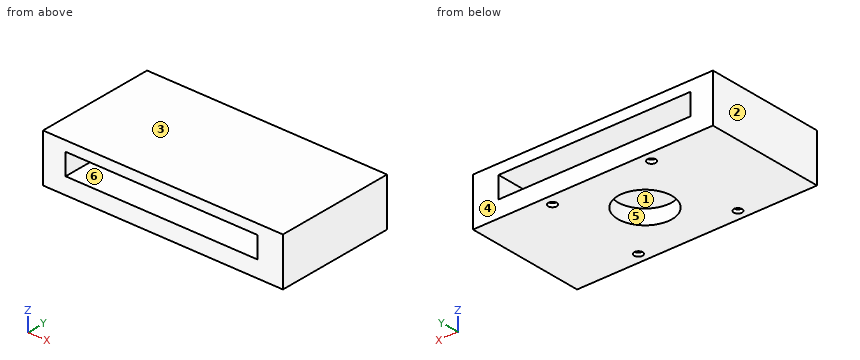
```python
from build123d import *

# Parameters (mm, degrees)
F0_W     = 2000
F0_H     = 425
F0_W_2   = 1598.0344712734
F0_H_2   = 178.1892329454
F1_DEPTH = 1000
F2_DEPTH = 25
F3_R     = 35
F4_DEPTH = 30
F5_R     = 225
F6_DEPTH = 122
F7_SCALE = 0.055


with BuildPart() as f1:
    # F0 (on Front) → F1 (new body)
    with BuildSketch(Plane.XZ):
        with Locations((-1000, 212.5)):
            Rectangle(F0_W, F0_H)
        with Locations((-1012.4687701464, 227.0783409476)):
            Rectangle(F0_W_2, F0_H_2, mode=Mode.SUBTRACT)
    extrude(amount=F1_DEPTH)

    # F2 (cut): a face of the model
    f2_faces = [f1.faces().sort_by_distance(p)[0] for p in [
        (-1000, -500, 425),
    ]]
    extrude(f2_faces, amount=-F2_DEPTH, mode=Mode.SUBTRACT)

    # F3 (on Top) → F4 (cut)
    with BuildSketch(Plane.XY):
        with Locations((-1415, -85)):
            Circle(F3_R)
        with Locations((-1415, -915)):
            Circle(F3_R)
        with Locations((-585, -915)):
            Circle(F3_R)
        with Locations((-585, -90)):
            Circle(F3_R)
    extrude(amount=F4_DEPTH, mode=Mode.SUBTRACT)

    # F5 (on face) → F6 (cut)
    with BuildSketch(Plane(origin=(0, 0, 0), x_dir=(1, 0, 0), z_dir=(0, 0, -1))):
        with Locations((-1000, 500)):
            Circle(F5_R)
    extrude(amount=-F6_DEPTH, mode=Mode.SUBTRACT)


with BuildPart() as f1_1:
    # F7: moved
    add(f1.part.scale(F7_SCALE))


solid = f1_1.part
```
The model under review builds one solid part; all positions refer to its coordinate system, in mm. Face numbers are marked on the shaded views. A direction names the side the tool comes from. Give positions to 0.01 mm unless a question says otherwise; leave off trailing zeros. Order: outer loops, then holes, each group sorted by start corner. A loop starts at its lowest first (then second) coordinate and runs counter-clockwise, first axis right, second up. Notation, with made-up numbers: (86, 71.5) - (116, 71.5) arc R24 ccw to (116, 103.5) - close; hole circle Ø10 at (10.5, -25). An arc over 180 degrees is marked (long way). Use CSV: the item, a comma, the result in double quotes. Start each with the question number.
Q1. Clearance check with flat-ended pins moving along their axes: pin 1 Ø1.2 at (x, y) = (-33, -49.5) entering from -Z; pin 2 Ø1.5 at (x, z) = (-22.5, 15) entering from +Y; pin 3 Ø7.5 at (x, y) = (-49.5, -30) entering from -Z. State where each tip first meets the part, or that it passes through.
Q2. We need section D-D, the plane y = -45.5. Write out the cut boundary in (x, z).
Q3. To check wall thickness, follow line 1 along Z through (x, y) = (-44, -17.5); line 2 along X through (y, z) = (-4.95, 0.75); line 3 along X through (y, z) = (-19, 17.25). State the ranges of each line that lie inside material, in increasing order. Write a range as [from, to].
Q4. We need section B-B, the plane z = 10.75. Write out the cut boundary in (x, y), and give its area (3 significant figures).
Q5. We need section A-A, the plane x = -55. Write out the cut boundary in (y, z) (3 decimals).
Q6. We need section C-C, the plane z = 4. Write out the cut boundary in (x, y) (3 decimals), and give its area (3 significant figures).
Q7. The part is to be moulded in two halves that separate along X. For the marked faces 1, 2 and 3, say which applies: +X half, -X half, draft (parallel to the pull), parting line (faces both ways), or undercut.
Q8. Tool access review of the marked faces 4, 5 and 6: name each direction out of +Z, -Z, +X, -X, +Y, -Y from which nothing blocks a thin tool from reaching the whole face with its end or side.
Outcome:
1,pin 1,"stops at z = 1.65"
1,pin 2,"passes through"
1,pin 3,"stops at z = 6.71"
2,outline,"(-110, 0) - (0, 0) - (0, 22) - (-110, 22) - close; hole (-99.63, 7.59) - (-11.74, 7.59) - (-11.74, 17.39) - (-99.63, 17.39) - close"
3,line 1,"z = [0, 7.59], [17.39, 22]"
3,line 2,"x = [-110, -79.73], [-75.92, -34.1], [-30.25, 0]"
3,line 3,"x = [-110, -99.63], [-11.74, 0]"
4,outline,"(-110, -55) - (-99.63, -55) - (-99.63, 0) - (-110, 0) - close; (-11.74, -55) - (0, -55) - (0, 0) - (-11.74, 0) - close"
4,area,"1,220 mm^2"
5,outline,"(-55, 0) - (-39.875, 0) - (-39.875, 6.71) - (-15.125, 6.71) - (-15.125, 0) - (0, 0) - (0, 7.589) - (-55, 7.589) - close; (-55, 17.39) - (0, 17.39) - (0, 22) - (-55, 22) - close"
6,outline,"(-110, -55) - (0, -55) - (0, 0) - (-110, 0) - close; hole circle Ø24.75 at (-55, -27.5)"
6,area,"5,570 mm^2"
7,face 1,"undercut"
7,face 2,"-X half"
7,face 3,"draft"
8,face 4,"+Z, -Z, +X, -X, +Y"
8,face 5,"-Z"
8,face 6,"+Y, -Y"
